Here's how the part is built. I have some questions about the finished solid (model axes, mm). A direction names the side the tool comes from. Round coordinates to 2 decimals unless told otherwise and drop trailing zeros. Write each loop counter-clockwise with the first axis right and the second up, starting at its lowest first coordinate (ties: lowest second). Pieces come first, ordered by that corner, then holes. Notation, with made-up numbers: (-36, 89.5) -> (-21, 89.5) arc R6 ccw to (-21, 93.5) -> close; hole circle Ø7 at (46.5, 82.25). An arc over 180 degrees is marked (long way). Put each result on its own line as item: value. Start each with the question number.
1. Suppose I cut it at C-C (x = -10.5). Please give me the cut outline in (y, z).
2. We'd pull the mould along Z, two halves only. Please class faces 1 (the face through (0.596, 2.815, -25.952)), 2 (the face through (0, 19, -9)), 3 (the face through (-23.977, 12.818, 1.055)), 4 (the face through (8.41, 17.255, 26.707)): +Z half, -Z half, draft (parallel to the pull), parting line (faces both ways), or undercut.
3. For pin 1 (8 mm diameter, centred on x = 17.5, y = 23, fed in from -Z); pin 2 (1.3 mm diameter, centred on y = 110, z = 4, fed in from +X); pin 3 (6 mm diameter, centred on x = 22, y = 37, fed in from -Z); pin 4 (3.5 mm diameter, centred on x = 0, y = 5.5, fed in from -Z), each with a flat end and sliding along its axis, tell me the tip position at first contact or that it passes through.
4. Suppose I cut it at D-D (y = 29.5). Please give me the cut outline in (x, z).
5. Which directions (+Z, -Z, +X, -X, +Y, -Y) give clear straight access to the entire face, cutting with the end or side of a thin tool? Please do faces 5 (the face through (-2.681, 54.72, 6.466)), 6 (the face through (4, 15, 0)), 7 (the face through (5, 26, 6)), 8 (the face through (0, 30, 23)).
6. Suppose I cut it at B-B (y = 5.5). Please give me the cut outline in (x, z).
7. I need wall thicknesses on probe 1 along Y at (x, z) = (0, 25); probe 2 along Y at (x, z) = (6, 9); probe 3 along Z at (x, y) = (3, 25.5). Which ranges of each line are inside material? Lowest first, please. Write a range as from..to.
8. Suppose I cut it at A-A (z = 12). Please give me the cut outline in (x, y).
```python
from build123d import *

# Parameters (mm, degrees)
F4_DEPTH  = 2
F5_R      = 24
F6_DEPTH  = 26
F7_R      = 7.5
F8_DEPTH  = 11
F9_R      = 20
F10_DEPTH = 4
F13_D     = 5.5
F14_R     = 2.5
F15_DEPTH = 5
F17_D     = 5
F17_DEPTH = 18
F17_TIP   = 1.5021515476


with BuildPart() as f1:
    # F0 (on Right) → F1 (revolve)
    with BuildSketch(Plane.YZ):
        Polygon((0, 28), (0, 0), (133, 0), (133, 5.5), (75, 5.5), (75, 7), (35, 7), (35, 28), align=None)
    revolve(axis=Axis((0, 66.5, 0), (0, 1, 0)))

    # F3 (on offset) → F4 (cut)
    with BuildSketch(Plane.XY.offset(5.5)):
        with BuildLine():
            Line((0, 99), (0.5, 99))
            ThreePointArc((0.5, 99), (1.5606601718, 99.4393398282), (2, 100.5))
            Line((2, 100.5), (2, 133))
            Line((2, 133), (-2, 133))
            Line((-2, 133), (-2, 101))
            ThreePointArc((-2, 101), (-1.4142135624, 99.5857864376), (0, 99))
        make_face()
    extrude(amount=-F4_DEPTH, mode=Mode.SUBTRACT)

    # F5 (on face) → F6 (cut)
    with BuildSketch(Plane.XZ):
        Circle(F5_R)
    extrude(amount=-F6_DEPTH, mode=Mode.SUBTRACT)

    # F7 (on face) → F8 (join)
    with BuildSketch(Plane.XZ.offset(-26)):
        Circle(F7_R)
    extrude(amount=F8_DEPTH)

    # F9 (on face) → F10 (join)
    with BuildSketch(Plane.XZ.offset(-15)):
        Circle(F9_R)
    extrude(amount=-F10_DEPTH)

    # F13 (through all)
    with Locations(Plane.XY.offset(28)):
        with Locations((0, 5.5)):
            Hole(F13_D / 2)

    # F14 (on offset) → F15 (cut)
    with BuildSketch(Plane.XY.offset(28)):
        with Locations((0, 29.5)):
            Circle(F14_R)
    extrude(amount=-F15_DEPTH, mode=Mode.SUBTRACT)

    # F17
    with Locations(Plane.XZ.offset(-15)):
        with Locations((0, 0)):
            Hole(F17_D / 2, depth=F17_DEPTH)
            with Locations((0, 0, -(F17_DEPTH + F17_TIP / 2))):  # 118° drill point
                Cone(0, F17_D / 2, F17_TIP, mode=Mode.SUBTRACT)


solid = f1.part
```
Verdict:
1. outline: (0, -25.96) -> (35, -25.96) -> (35, 25.96) -> (0, 25.96) -> (0, 21.58) -> (26, 21.58) -> (26, -21.58) -> (0, -21.58) -> close; (15, -17.02) -> (19, -17.02) -> (19, 17.02) -> (15, 17.02) -> close
2. face 1: draft
2. face 2: undercut
2. face 3: undercut
2. face 4: parting line
3. pin 1: stops at z = -24.53
3. pin 2: stops at x = 4.36
3. pin 3: stops at z = -19.83
3. pin 4: passes through
4. outline: (-2.5, 23) -> (-2.5, 27.89) arc R28 ccw (long way) to (2.5, 27.89) -> (2.5, 23) -> close; hole circle Ø5 at (0, 0)
5. face 5: +Y
5. face 6: -Y
5. face 7: none
5. face 8: +Z
6. outline: (-2.75, -27.86) -> (-2.75, -23.84) arc R24 cw to (-2.75, 23.84) -> (-2.75, 27.86) arc R28 ccw to start; (2.75, -27.86) arc R28 ccw to (2.75, 27.86) -> (2.75, 23.84) arc R24 cw to (2.75, -23.84) -> close
7. probe 1: y = 0..2.75, 8.25..27, 32..35
7. probe 2: y = 15..19, 26..35
7. probe 3: z = -27.84..-23.81, -6.87..6.87, 23.81..27.84
8. outline: (-25.3, 0) -> (-20.78, 0) -> (-20.78, 26) -> (20.78, 26) -> (20.78, 0) -> (25.3, 0) -> (25.3, 35) -> (-25.3, 35) -> close; (-16, 15) -> (16, 15) -> (16, 19) -> (-16, 19) -> close
